Model file for the job. Use its own axes, mm. A direction names the side the tool comes from. Round coordinates to 2 decimals unless told otherwise and drop trailing zeros. Loops run counter-clockwise (first coordinate to the right, second up) from the corner with the lowest first, then second, coordinate; pieces in that order, holes last. Notation, with made-up numbers: (-35.75, 55) - (17.25, 55) arc R29 cw to (17.25, 88) - close; hole circle Ø5 at (23, 21.5). An arc over 180 degrees is marked (long way). Answer as a JSON object with one key per item and string values.
from build123d import *

# Parameters (mm, degrees)
SKETCH1_W            = 35
SKETCH1_H            = 40.6
BOSS_EXTRUDE1_DEPTH  = 18
SCALE1_SCALE         = 1.15
SKETCH7_W            = 35
SKETCH7_H            = 40.6
CUT_EXTRUDE1_DEPTH   = 15
FILLET1_R            = 10
FILLET2_R            = 5
FILLET3_R            = 1
FILLET4_R            = 1
SKETCH9_R            = 11.5
CUT_EXTRUDE2_DEPTH   = 72.03051567
CHAMFER1_SIZE        = 2
SWEEP1_PROFILE_R     = 13.75
CUT_SWEEP2_PROFILE_R = 11.5
SKETCH13_W           = 4.429427916
SKETCH13_H           = 5.487691531
CUT_EXTRUDE3_DEPTH   = 10
SKETCH34_W           = 2.806069431
SKETCH34_H           = 2.063682343
CUT_EXTRUDE6_DEPTH   = 2


with BuildPart() as part:
    # Sketch1 → Boss-Extrude1 (new body)
    with BuildSketch(Plane.YZ):
        with Locations((-17.5, -20.3)):
            Rectangle(SKETCH1_W, SKETCH1_H)
        Polygon((-47, -12.8), (-47, -27.8), (-35, -40.6), (-35, 0), align=None)
        with BuildLine():
            Line((25.653410767, -24.537854564), (0, -40.6))
            Line((0, -40.6), (0, 0))
            Line((0, 0), (25.653410767, -16.062145436))
            ThreePointArc((25.653410767, -16.062145436), (28, -20.3), (25.653410767, -24.537854564))
        make_face()
    extrude(amount=BOSS_EXTRUDE1_DEPTH)


with BuildPart() as part_1:
    # Scale1: scaled about (9, -13.156905102, -20.3)
    add(part.part.scale(SCALE1_SCALE).moved(Location((-1.35, 1.973535765, 3.045))))

    # Sketch7 → Cut-Extrude1 (cut)
    with BuildSketch(Plane.YZ.offset(19.35)):
        with Locations((-18.076464235, -20.3)):
            Rectangle(SKETCH7_W, SKETCH7_H)
        Polygon((-47.576464235, -12.8), (-47.576464235, -27.8), (-35.576464235, -40.6), (-35.576464235, 0), align=None)
        with BuildLine():
            Line((25.076946532, -24.537854564), (-0.576464235, -40.6))
            Line((-0.576464235, -40.6), (-0.576464235, 0))
            Line((-0.576464235, 0), (25.076946532, -16.062145436))
            ThreePointArc((25.076946532, -16.062145436), (27.423535765, -20.3), (25.076946532, -24.537854564))
        make_face()
    extrude(amount=-CUT_EXTRUDE1_DEPTH, mode=Mode.SUBTRACT)

    # Fillet1
    fillet1_edges = [part_1.edges().sort_by_distance(p)[0] for p in [
        (9, 1.973535765, 3.045),
        (9, 1.973535765, -43.645),
        (9, -38.276464235, -43.645),
        (9, -52.076464235, -28.925),
        (9, -52.076464235, -11.675),
        (9, -38.276464235, 3.045),
    ]]
    fillet(fillet1_edges, radius=FILLET1_R)

    # Fillet2
    fillet2_edges = [part_1.edges().sort_by_distance(p)[0] for p in [
        (11.85, -35.576464235, 0),
        (11.85, -0.576464235, 0),
        (11.85, -0.576464235, -40.6),
        (11.85, -35.576464235, -40.6),
        (11.85, -47.576464235, -27.8),
        (11.85, -47.576464235, -12.8),
    ]]
    fillet(fillet2_edges, radius=FILLET2_R)

    # Fillet3
    fillet3_edges = [part_1.edges().sort_by_distance(p)[0] for p in [
        (19.35, 17.941495924, -33.647120938),
        (19.35, 34.173535765, -20.3),
        (19.35, -17.421465972, 3.045),
        (19.35, 17.941495924, -6.952879062),
        (19.35, -45.305676214, -4.452826111),
        (19.35, -52.076464235, -20.3),
        (19.35, -45.305676214, -36.147173889),
        (19.35, -17.421465972, -43.645),
        (19.35, -37.919435742, -42.820895403),
        (19.35, 1.861910332, -43.256375845),
        (19.35, -51.375757767, -28.647907393),
        (19.35, -51.375757767, -11.952092607),
        (19.35, -37.919435742, 2.220895403),
        (19.35, 1.861910332, 2.656375845),
    ]]
    fillet(fillet3_edges, radius=FILLET3_R)

    # Fillet4
    fillet4_edges = [part_1.edges().sort_by_distance(p)[0] for p in [
        (-1.35, 34.173535765, -20.3),
        (-1.35, 17.941495924, -33.647120938),
        (-1.35, -17.421465972, 3.045),
        (-1.35, 17.941495924, -6.952879062),
        (-1.35, -17.421465972, -43.645),
        (-1.35, -45.305676214, -36.147173889),
        (-1.35, -52.076464235, -20.3),
        (-1.35, -45.305676214, -4.452826111),
        (-1.35, -37.919435742, -42.820895403),
        (-1.35, 1.861910332, -43.256375845),
        (-1.35, -51.375757767, -28.647907393),
        (-1.35, -51.375757767, -11.952092607),
        (-1.35, -37.919435742, 2.220895403),
        (-1.35, 1.861910332, 2.656375845),
    ]]
    fillet(fillet4_edges, radius=FILLET4_R)

    # Sketch9 → Cut-Extrude2 (cut, through all)
    with BuildSketch(Plane(origin=(-1.35, 0, 0), x_dir=(0, -1, 0), z_dir=(-1, 0, 0))):
        with Locations(Location((8.54339023, -20.3, 0), (0, 0, 90))):
            Circle(SKETCH9_R)
    extrude(amount=-CUT_EXTRUDE2_DEPTH, mode=Mode.SUBTRACT)

    # Chamfer1
    chamfer1_edges = [part_1.edges().sort_by_distance(p)[0] for p in [
        (4.35, -8.54339023, -31.8),
    ]]
    chamfer(chamfer1_edges, length=CHAMFER1_SIZE)

    # Sweep1: sweep along a path in Sketch11
    with BuildLine(Plane.XY.offset(-20.3)) as sweep1_path:
        Line((-1.35, -8.54339023), (-41.35, -8.54339023))
        ThreePointArc((-41.35, -8.54339023), (-55.492135624, -14.401254607), (-61.35, -28.54339023))
        Line((-61.35, -28.54339023), (-61.35, -88.54339023))
    # Sweep1 profile (on start of the path) → Sweep1 (sweep)
    with BuildSketch(Plane(origin=(-1.35, -8.54339023, -20.3), x_dir=(0, -1, 0), z_dir=(-1, 0, 0))):
        Circle(SWEEP1_PROFILE_R)
    sweep(path=sweep1_path.line)

    # Cut-Sweep2: sweep along a path in Sketch11_3
    with BuildLine(Plane.XY.offset(-20.3)) as cut_sweep2_path:
        Line((-1.35, -8.54339023), (-41.35, -8.54339023))
        ThreePointArc((-41.35, -8.54339023), (-55.492135624, -14.401254607), (-61.35, -28.54339023))
        Line((-61.35, -28.54339023), (-61.35, -88.54339023))
    # Cut-Sweep2 profile (on start of the path) → Cut-Sweep2 (sweep, cut)
    with BuildSketch(Plane(origin=(-1.35, -8.54339023, -20.3), x_dir=(0, -1, 0), z_dir=(-1, 0, 0))):
        Circle(CUT_SWEEP2_PROFILE_R)
    sweep(path=cut_sweep2_path.line, mode=Mode.SUBTRACT)

    # Sketch13 → Cut-Extrude3 (cut)
    with BuildSketch(Plane.XZ.offset(88.54339023)):
        with Locations((-61.35, -30.148697086)):
            Rectangle(SKETCH13_W, SKETCH13_H)
    extrude(amount=-CUT_EXTRUDE3_DEPTH, mode=Mode.SUBTRACT)

    # Sketch34 → Cut-Extrude6 (cut)
    with BuildSketch(Plane.YZ.offset(-63.564713958)):
        with Locations((-79.980636632, -31.987266617)):
            Rectangle(SKETCH34_W, SKETCH34_H)
    extrude(amount=-CUT_EXTRUDE6_DEPTH, mode=Mode.SUBTRACT)


solid = part_1.part
1) Probe probe 1 along X at (y, z) = (-34.5, -21); probe 2 along Z at (x, y) = (-61.35, -61); probe 3 along X at (y, z) = (4.5, -34.5). List the from-to ranges inside material, lowest first.
Values follow:
{"probe 1": "-75.08 to -72.83, -49.87 to -47.62, -1.35 to 4.35", "probe 2": "-34.05 to -31.8, -8.8 to -6.55", "probe 3": "-1.35 to 4.35"}
2) Tool access for faces 4 (the cylindrical face through (-19.81, -13.97, -10.16)), 5 (the cylindrical face through (9.131, -51.356, -28.697)), 6 (the cylindrical face through (9.131, -51.395, -12.001)), 7 (the cylindrical face through (-1.05, -45.04, -4.59)): list every direction of +Z, -Z, +X, -X, +Y, -Y with a clear straight run to the whole face (end or side of a thin tool).
Values follow:
{"face 4": "+X", "face 5": "-Z, +X, -Y", "face 6": "+Z, +X, -Y", "face 7": "+Z, -Y"}
3) Slice it at B-B on x = -32. List the corners of the cut face in (y, z).
Values follow:
{"outline": "circle Ø27.5 at (-8.54, -20.3); hole circle Ø23 at (-8.54, -20.3)"}
4) Two-plate mould, pull along X, no slides. Class faces 1 (the cylindrical face through (9.13, 1.82, -43.27)), 2 (the cylindrical face through (-1.049, -45.155, -35.891)), 3 (the cylindrical face through (-1.049, 17.601, -33.524)): pulls with the +X half, pulls with the -X half, needs draft (parallel to the pull), parting line crosses it, or undercut.
Values follow:
{"face 1": "needs draft", "face 2": "undercut", "face 3": "pulls with the -X half"}
5) Drop flat-ended pins along their axis: P1, Ø1.5, axis at x = -50.5, z = -7.5, coming from the +Y side; P2, Ø14, axis at x = -61.35, z = -20.3, coming from the -Y side; P3, Ø5.5, axis at x = 15.5, z = -22.5, coming from the +Y side; P4, Ø3.5, axis at x = -61, y = -82, coming from the +Z side. Give the stop position or say it passes through.
Values follow:
{"P1": "y = -3.52", "P2": "y = -12.32", "P3": "y = 34.17", "P4": "z = -6.55"}
